from build123d import *

# Parameters (mm, degrees)
F0_W     = 88.9
F0_H     = 38.1
F1_DEPTH = 50.8
F2_W     = 50.8
F2_H     = 25.4
F3_DEPTH = 50.801
F4_W     = 38.1
F4_H     = 25.4
F5_DEPTH = 38.101
F6_R     = 6.35
F7_DEPTH = 12.701


with BuildPart() as f1:
    # F0 (on Front) → F1 (new body)
    with BuildSketch(Plane.XZ):
        Rectangle(F0_W, F0_H)
    extrude(amount=F1_DEPTH)

    # F2 (on face) → F3 (cut, through all)
    with BuildSketch(Plane.XZ.offset(50.8)):
        with Locations((-0.658147, 6.35)):
            Rectangle(F2_W, F2_H)
    extrude(amount=-F3_DEPTH, mode=Mode.SUBTRACT)

    # F4 (on face) → F5 (cut, through all)
    with BuildSketch(Plane.XY.offset(19.05)):
        with Locations((25.4, -38.1)):
            Rectangle(F4_W, F4_H)
    extrude(amount=-F5_DEPTH, mode=Mode.SUBTRACT)

    # F6 (on face) → F7 (cut, through all)
    with BuildSketch(Plane.XY.offset(-6.35)):
        with Locations((6.35, -12.7)):
            Circle(F6_R)
        with Locations((-19.05, -38.1)):
            Circle(F6_R)
    extrude(amount=-F7_DEPTH, mode=Mode.SUBTRACT)


solid = f1.part
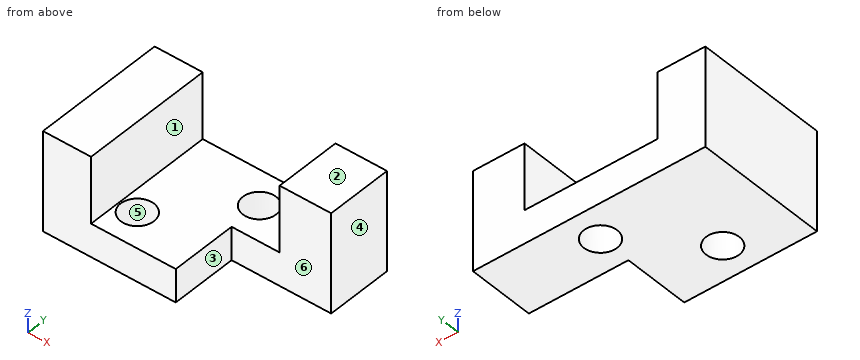
Could you check a few things on this model? Use its own coordinates, in mm. Face numbers are marked on the shaded views. A direction names the side the tool comes from. Coordinates: 2 decimals unless noted, no trailing zeros. Loops run counter-clockwise (first coordinate to the right, second up) from the corner with the lowest first, then second, coordinate; pieces in that order, holes last.
1. For P1, Ø11.5, axis at x = 29, z = -2.5, coming from the -Y side; P2, Ø10, axis at x = -19.05, y = -38.1, coming from the -Z side; P3, Ø4, axis at y = -37.5, z = -12.5, coming from the +X side; P4, Ø4, axis at y = -33, z = 4.5, coming from the +X side, each with a flat end and sliding along its axis, tell me the tip position at first contact or that it passes through.
2. Imagine slicing it at C-C (x = -19.05). Please give me the cut outline in (y, z).
3. I need wall thicknesses on L1, parallel to Y at x = -19, z = -12; L2, parallel to X at y = -13.5, z = 12; L3, parallel to Y at x = 6, z = -9. Which ranges of each line are inside material? Lowest first, please.
4. Imagine slicing it at B-B (y = -38.1). Please give me the cut outline in (x, z), and give its area (3 significant figures).
5. For the marked faces 1, 2 and 3, which set-ups out of +Z, -Z, +X, -X, +Y, -Y let a thin tool reach every point of the face, with its end or its side?
6. Imagine slicing it at A-A (z = 0.5). Please give me the cut outline in (x, y).
7. Imagine slicing it at D-D (z = -11.5). Please give me the cut outline in (x, y), and give its area (3 significant figures).
8. We'd pull the mould along Y, two halves only. Please class the marked faces 4, 5 and 6: released by +Y, released by -Y, zero draft, split by the parting line, or undercut.
Computed values:
1. P1: stops at y = -25.4
1. P2: passes through
1. P3: stops at x = 6.35
1. P4: stops at x = -26.06
2. outline: (-50.8, -19.05) - (-44.45, -19.05) - (-44.45, -6.35) - (-50.8, -6.35) - close; (-31.75, -19.05) - (0, -19.05) - (0, -6.35) - (-31.75, -6.35) - close
3. L1: y = -50.8 to -44.45, -31.75 to 0
3. L2: x = -44.45 to -26.06, 24.74 to 44.45
3. L3: y = -50.8 to -19.04, -6.36 to 0
4. outline: (-44.45, -19.05) - (-25.4, -19.05) - (-25.4, -6.35) - (-26.06, -6.35) - (-26.06, 19.05) - (-44.45, 19.05) - close; (-12.7, -19.05) - (6.35, -19.05) - (6.35, -6.35) - (-12.7, -6.35) - close
4. area: 951 mm2
5. face 1: +Z, +Y, -Y
5. face 2: +Z, +X, -X, +Y, -Y
5. face 3: +Z, -Z, +X, -Y
6. outline: (-44.45, -50.8) - (-26.06, -50.8) - (-26.06, 0) - (-44.45, 0) - close; (24.74, -25.4) - (44.45, -25.4) - (44.45, 0) - (24.74, 0) - close
7. outline: (-44.45, -50.8) - (6.35, -50.8) - (6.35, -25.4) - (44.45, -25.4) - (44.45, 0) - (-44.45, 0) - close; hole circle Ø12.7 at (-19.05, -38.1); hole circle Ø12.7 at (6.35, -12.7)
7. area: 3,300 mm2
8. face 4: zero draft
8. face 5: undercut
8. face 6: released by -Y
